Could you check a few things on this model? Use its own coordinates, in mm. A direction names the side the tool comes from. Coordinates: 2 decimals unless noted, no trailing zeros. Loops run counter-clockwise (first coordinate to the right, second up) from the corner with the lowest first, then second, coordinate; pieces in that order, holes last. Notation, with made-up numbers: M -17,-24 L 17,-24 A17 ccw 17,0 Z; hole C 47.25,27 d3. An arc over 180 degrees is marked long. Use one line per item in the form item = value. Start each with the question number.
```python
from build123d import *

# Parameters (mm, degrees)
SKETCH1_W            = 25
SKETCH1_H            = 20
BOSS_EXTRUDE1_DEPTH  = 3
SKETCH2_W            = 3
SKETCH2_H            = 20
BOSS_EXTRUDE2_DEPTH  = 40
SKETCH6_W            = 45
SKETCH6_H            = 20
BOSS_EXTRUDE3_DEPTH  = 3
SKETCH9_W            = 3
SKETCH9_H            = 20
BOSS_EXTRUDE4_DEPTH  = 40
CHAMFER1_SIZE        = 6
SKETCH17_W           = 14.8
SKETCH17_H           = 14.8
SKETCH17_W_2         = 10.8
SKETCH17_H_2         = 10.8
BOSS_EXTRUDE7_DEPTH  = 10
SKETCH18_W           = 14.8
SKETCH18_H           = 14.8
BOSS_EXTRUDE8_DEPTH  = 2
SKETCH21_W           = 14.8
SKETCH21_H           = 14.8
BOSS_EXTRUDE11_DEPTH = 2
BOSS_EXTRUDE12_REACH = 89.482
BOSS_EXTRUDE13_DEPTH = 7.6
CHAMFER4_SIZE        = 17
CHAMFER4_SIZE_2      = 9.039060338
CUT_EXTRUDE8_DEPTH   = 13
SKETCH27_W           = 2
SKETCH27_H           = 10.8
CUT_EXTRUDE10_DEPTH  = 3
CUT_EXTRUDE12_DEPTH  = 10
CUT_EXTRUDE13_START  = -10
CUT_EXTRUDE13_DEPTH  = 10
SKETCH40_W           = 2
SKETCH40_H           = 10.8
CUT_EXTRUDE16_DEPTH  = 2
SKETCH41_W           = 2
SKETCH41_H           = 10.8
CUT_EXTRUDE17_DEPTH  = 2
SKETCH51_W           = 3
SKETCH51_H           = 20
BOSS_EXTRUDE14_DEPTH = 64
SKETCH50_R           = 1.5
CUT_EXTRUDE22_DEPTH  = 82.203258526


# Read off the part's stored shape, not the designer's step: Mirror3
with BuildPart() as part:
    # Sketch1 → Boss-Extrude1 (new body)
    with BuildSketch(Plane.XY):
        Rectangle(SKETCH1_W, SKETCH1_H)
    extrude(amount=BOSS_EXTRUDE1_DEPTH)

    # Sketch2 → Boss-Extrude2 (add)
    with BuildSketch(Plane.XY.offset(3)):
        with Locations((-11, 0)):
            Rectangle(SKETCH2_W, SKETCH2_H)
    extrude(amount=BOSS_EXTRUDE2_DEPTH)

    # Sketch6 → Boss-Extrude3 (add)
    with BuildSketch(Plane(origin=(0, 0, 0), x_dir=(-1, 0, 0), z_dir=(0, 0, -1))):
        with Locations((-35, 0)):
            Rectangle(SKETCH6_W, SKETCH6_H)
    extrude(amount=-BOSS_EXTRUDE3_DEPTH)

    # Sketch9 → Boss-Extrude4 (add)
    with BuildSketch(Plane.XY.offset(3)):
        with Locations((56, 0)):
            Rectangle(SKETCH9_W, SKETCH9_H)
    extrude(amount=BOSS_EXTRUDE4_DEPTH)

    # Chamfer1
    chamfer1_edges = [part.edges().sort_by_distance(p)[0] for p in [
        (-11, -10, 43),
        (-11, 10, 43),
        (56, -10, 43),
        (56, 10, 43),
    ]]
    chamfer(chamfer1_edges, length=CHAMFER1_SIZE)

    # Sketch17 → Boss-Extrude7 (add)
    # profile 1 of 2: a face of its own
    with BuildSketch(Plane(origin=(57.5, 0, 0), x_dir=(0, 0, -1), z_dir=(1, 0, 0))):
        with Locations((3.445401219, -5)):
            Rectangle(SKETCH17_W, SKETCH17_H)
        with Locations((3.445401219, -5)):
            Rectangle(SKETCH17_W_2, SKETCH17_H_2, mode=Mode.SUBTRACT)
    # profile 2 of 2: a face of its own
    with BuildSketch(Plane(origin=(57.5, 0, 0), x_dir=(0, 0, -1), z_dir=(1, 0, 0))):
        with Locations((-36.004598781, -5)):
            Rectangle(SKETCH17_W, SKETCH17_H)
        with Locations((-36.004598781, -5)):
            Rectangle(SKETCH17_W_2, SKETCH17_H_2, mode=Mode.SUBTRACT)
    extrude(amount=BOSS_EXTRUDE7_DEPTH)

    # Sketch18 → Boss-Extrude8 (add)
    with BuildSketch(Plane.ZY.offset(-57.5)):
        with Locations((-3.445401219, -5)):
            Rectangle(SKETCH18_W, SKETCH18_H)
    extrude(amount=BOSS_EXTRUDE8_DEPTH)

    # Sketch21 → Boss-Extrude11 (add)
    with BuildSketch(Plane.ZY.offset(-57.5)):
        with Locations((36.004598781, -5)):
            Rectangle(SKETCH21_W, SKETCH21_H)
    extrude(amount=BOSS_EXTRUDE11_DEPTH)

    # Boss-Extrude12: up to this face of the body (flat: up to its plane)
    boss_extrude12_end = Plane(part.part.faces().sort_by_distance((62.311518325, -5.194764398, 28.604598781))[0])
    # Sketch22 → Boss-Extrude12 (add, up to the picked face)
    with BuildSketch(Plane.XY.offset(43.404598781), mode=Mode.PRIVATE) as boss_extrude12_sk1:
        Polygon((57.5, 2.4), (57.5, 10), (67.5, 2.4), align=None)
    boss_extrude12_tool1 = split(extrude(boss_extrude12_sk1.sketch, amount=-BOSS_EXTRUDE12_REACH, mode=Mode.PRIVATE), bisect_by=boss_extrude12_end, keep=Keep.BOTH, mode=Mode.PRIVATE)
    add(boss_extrude12_tool1.solids().sort_by(Axis((60.833333, 4.933333, 43.404599), (0, 0, -1)))[0])

    # Sketch23 → Boss-Extrude13 (add)
    with BuildSketch(Plane(origin=(0, 2.4, 0), x_dir=(1, 0, 0), z_dir=(0, 1, 0))):
        Polygon((55.5, 0), (57.5, 0), (57.5, -3.954598781), (67.5, -3.954598781), (67.5, 10.492881323), (67.147480104, 10.845401219), (55.5, 10.845401219), align=None)
    extrude(amount=BOSS_EXTRUDE13_DEPTH)

    # Chamfer4
    # the kernel refuses this chamfer: 17, 9.039060338 mm, written as the material it adds along each edge
    # the kernel refuses this chamfer: 17, 9.039060338 mm, written as the material it takes off along each edge
    with BuildSketch(Plane(origin=(98.618530871, 10, 20.625649548), x_dir=(-0.7069904920950609, 0.018135274312576832, 0.706990492095043), z_dir=(-0.7071067811865386, 0, -0.7071067811865565))) as chamfer4_2_piece_1_section:
        Polygon((CHAMFER4_SIZE * 0.99983554239, -CHAMFER4_SIZE * 0.0181352743126), (-CHAMFER4_SIZE_2 * 0.0181352743131, -CHAMFER4_SIZE_2 * 0.999835542417), (0, 0), align=None)
    chamfer4_2_piece_1 = extrude(amount=88.515035216, mode=Mode.PRIVATE)
    chamfer4_2_piece_1 = split(chamfer4_2_piece_1, bisect_by=Plane(origin=(63.588119048, 2.4, 1.757393484), z_dir=(0, 1, 0)), keep=Keep.TOP, mode=Mode.PRIVATE)
    add(chamfer4_2_piece_1, mode=Mode.SUBTRACT)

    # Sketch24 → Cut-Extrude8 (cut)
    with BuildSketch(Plane.ZY.offset(-57.5)):
        Polygon((37, 10), (43.404598781, 10), (43.404598781, 2.4), (43, 2.4), (43, 4), align=None)
    extrude(amount=-CUT_EXTRUDE8_DEPTH, mode=Mode.SUBTRACT)

    # Mirror3
    split(bisect_by=Plane.ZY.offset(-22.5), keep=Keep.BOTTOM)

    # Mirror3 2: part across plane


with BuildPart() as part_1:
    add(part.part)
    add(part.part.mirror(Plane.ZY.offset(-22.5)))

    # Sketch27 → Cut-Extrude10 (cut)
    with BuildSketch(Plane.ZY.offset(22.5)):
        with Locations((2.954598781, -5)):
            Rectangle(SKETCH27_W, SKETCH27_H)
    cut_extrude10 = extrude(amount=-CUT_EXTRUDE10_DEPTH, mode=Mode.SUBTRACT)

    # Mirror4: Cut-Extrude10 across plane
    add(cut_extrude10.mirror(Plane.ZY.offset(-22.5)), mode=Mode.SUBTRACT)

    # Sketch32 → Cut-Extrude12 (cut)
    with BuildSketch(Plane(origin=(0, 0, -10.845401219), x_dir=(-1, 0, 0), z_dir=(0, 0, -1))):
        with BuildLine():
            Line((19.790168373, -6.5), (17.5, -6.5))
            ThreePointArc((17.5, -6.5), (16, -5), (17.5, -3.5))
            Line((17.5, -3.5), (19.790168373, -3.5))
            ThreePointArc((19.790168373, -3.5), (21.290168373, -5), (19.790168373, -6.5))
        make_face()
        with BuildLine():
            Line((-64.790168373, -6.5), (-62.5, -6.5))
            ThreePointArc((-62.5, -6.5), (-61, -5), (-62.5, -3.5))
            Line((-62.5, -3.5), (-64.790168373, -3.5))
            ThreePointArc((-64.790168373, -3.5), (-66.290168373, -5), (-64.790168373, -6.5))
        make_face()
    extrude(amount=-CUT_EXTRUDE12_DEPTH, mode=Mode.SUBTRACT)

    # Sketch33 → Cut-Extrude13 (cut)
    with BuildSketch(Plane.XY.offset(43.404598781).offset(CUT_EXTRUDE13_START)):
        with BuildLine():
            Line((62.5, -3.5), (64.5, -3.5))
            ThreePointArc((64.5, -3.5), (66, -5), (64.5, -6.5))
            Line((64.5, -6.5), (62.5, -6.5))
            ThreePointArc((62.5, -6.5), (61, -5), (62.5, -3.5))
        make_face()
        with BuildLine():
            Line((-17.5, -6.5), (-19.5, -6.5))
            ThreePointArc((-19.5, -6.5), (-21, -5), (-19.5, -3.5))
            Line((-19.5, -3.5), (-17.5, -3.5))
            ThreePointArc((-17.5, -3.5), (-16, -5), (-17.5, -6.5))
        make_face()
    extrude(amount=CUT_EXTRUDE13_DEPTH, mode=Mode.SUBTRACT)

    # Sketch40 → Cut-Extrude16 (cut)
    with BuildSketch(Plane(origin=(64.5, 0, 0), x_dir=(0, 0, -1), z_dir=(1, 0, 0))):
        with Locations((-2.954598781, -5)):
            Rectangle(SKETCH40_W, SKETCH40_H)
    extrude(amount=-CUT_EXTRUDE16_DEPTH, mode=Mode.SUBTRACT)

    # Sketch41 → Cut-Extrude17 (cut)
    with BuildSketch(Plane.ZY.offset(19.5)):
        with Locations((2.954598781, -5)):
            Rectangle(SKETCH41_W, SKETCH41_H)
    extrude(amount=-CUT_EXTRUDE17_DEPTH, mode=Mode.SUBTRACT)

    # Sketch51 → Boss-Extrude14 (add)
    with BuildSketch(Plane(origin=(-9.5, 0, 0), x_dir=(0, 0, -1), z_dir=(1, 0, 0))):
        with Locations((-35.5, 0)):
            Rectangle(SKETCH51_W, SKETCH51_H)
    extrude(amount=BOSS_EXTRUDE14_DEPTH)

    # Sketch50 → Cut-Extrude22 (cut, through all)
    with BuildSketch(Plane(origin=(0, 0, 0), x_dir=(-1, 0, 0), z_dir=(0, 0, -1))):
        with Locations(Location((5.5, 5, 0), (0, 0, 90))):
            Circle(SKETCH50_R)
        with Locations(Location((5.5, -5, 0), (0, 0, 90))):
            Circle(SKETCH50_R)
        with Locations(Location((-50.5, -5, 0), (0, 0, 90))):
            Circle(SKETCH50_R)
        with Locations(Location((-50.5, 5, 0), (0, 0, 90))):
            Circle(SKETCH50_R)
        with Locations(Location((-27.5, 5, 0), (0, 0, 90))):
            Circle(SKETCH50_R)
        with Locations(Location((-27.5, -5, 0), (0, 0, 90))):
            Circle(SKETCH50_R)
        with Locations(Location((-17.5, -5, 0), (0, 0, 90))):
            Circle(SKETCH50_R)
        with Locations(Location((-17.5, 5, 0), (0, 0, 90))):
            Circle(SKETCH50_R)
    extrude(amount=-CUT_EXTRUDE22_DEPTH, mode=Mode.SUBTRACT)


solid = part_1.part
```
Item 1: For faces 4 (the cylindrical face through (61, -5, -10)), 5 (the flat face through (-16, -4, 41.405)), 6 (the cylindrical face through (61, -5, 42)), 7 (the flat face through (22, 0, 34)), which set-ups out of +Z, -Z, +X, -X, +Y, -Y let a thin tool reach every point of the face, with its end or its side?
Item 2: I'm going to push flat-ended pins straight in: P1, Ø0.6, axis at x = 63.5, z = -9.5, coming from the +Y side; P2, Ø7.5, axis at y = -6, z = -1, coming from the -X side; P3, Ø0.6, axis at y = -5, z = 2.5, coming from the +X side; P4, Ø2.5, axis at x = 17.5, y = -5, coming from the -Z side. Where does each tip first touch, or does it pass through?
Item 3: I want a section at A-A (x = -5.5). Write out the boundary of the cut face in (y, z).
Item 4: I want a section at D-D (x = 56.5). Write out the boundary of the cut face in (y, z), plus the area to 3 significant figures.
Item 5: I want a section at B-B (x = 33.5). Write out the boundary of the cut face in (y, z).
Item 6: I want a section at C-C (y = -5.5). Count the separate pieces of the cut face and the enclosed holes in it, plus the area to 3 significant figures.
Item 7: Thinking about a two-plate mould opening in X: for faces 1 (the flat face through (61.08, 6.25, -2.84)), 2 (the flat face through (22, 0, 3)), 3 (the flat face through (62, 0.4, 36)), which applies, pulls with the +X half, pulls with the -X half, needs draft (parallel to the pull), parting line crosses it, or undercut?
Item 8: Please list where these lines run through material, in increasing order: line 1 along X through (y, z) = (5, 1.85); line 2 along X through (y, z) = (-5, 1.15); line 3 along X through (y, z) = (-6.5, 18).
Worked answers:
q1.face_4 = -Z
q1.face_5 = -X
q1.face_6 = +Z
q1.face_7 = +Y, -Y
q2.P1 = 3
q2.P2 = -17.5
q2.P3 = 62.5
q2.P4 = through
q3.outline = M -10,0 L -6.5,0 L -6.5,3 L -10,3 Z; M -10,34 L -6.5,34 L -6.5,37 L -10,37 Z; M -3.5,0 L 3.5,0 L 3.5,3 L -3.5,3 Z; M -3.5,34 L 3.5,34 L 3.5,37 L -3.5,37 Z; M 6.5,0 L 10,0 L 10,3 L 6.5,3 Z; M 6.5,34 L 10,34 L 10,37 L 6.5,37 Z
q4.outline = M -12.4,-10.85 L 4.96,-10.85 L 10,2.55 L 10,37 L 4,43 L 2.4,43 L 2.4,43.4 L -12.4,43.4 L -12.4,28.6 L -10,28.6 L -10,3.95 L -12.4,3.95 Z
q4.area = 1,100 mm²
q5.outline = M -10,0 L 10,0 L 10,3 L -10,3 Z; M -10,34 L 10,34 L 10,37 L -10,37 Z
q6.separate_pieces = 12
q6.enclosed_holes = 0
q6.area = 716 mm²
q7.face_1 = pulls with the +X half
q7.face_2 = undercut
q7.face_3 = needs draft
q8.line_1 = -22.5 to -7, -4 to 16, 19 to 26, 29 to 49, 52 to 67.5
q8.line_2 = -12.5 to -7, -4 to 16, 19 to 26, 29 to 49, 52 to 57.5
q8.line_3 = -12.5 to -9.5, 54.5 to 57.5
